For this review, take the finished solid that the model builds, in its own axes (mm). A direction names the side the tool comes from. Round coordinates to 2 decimals unless told otherwise and drop trailing zeros. Loops run counter-clockwise (first coordinate to the right, second up) from the corner with the lowest first, then second, coordinate; pieces in that order, holes last.
1) Insertion check: pin 1 (3 mm diameter, centred on y = 8, z = -0.5, fed in from +X); pin 2 (3 mm diameter, centred on x = 13.5, y = 3.5, fed in from -Z); pin 3 (8 mm diameter, centred on y = 15, z = -6, fed in from +X); pin 4 (1.5 mm diameter, centred on x = 1, y = 14, fed in from +Z). Each pin has a flat end and moves straight along its axis. Give the tip position at first contact, or say it passes through.
2) Take a section at B-B (z = 0). State the section outline as (x, y) points (3 decimals), then the cut area to 3 significant figures.
3) Take a section at C-C (y = 7.5). State the section outline as (x, z) points.
4) Wall thickness on L1, parallel to Y at x = 3.5, z = 7.25; L2, parallel to Y at x = 9.5, z = -3.25 (3 decimals); L3, parallel to X at y = 11.25, z = -1.75: over which ranges is each line inside the solid? List them lowest first.
5) Take a section at D-D (z = 2.5). State the section outline as (x, y) points (3 decimals).
6) Tool access review of faces 1 (the cylindrical face through (14.5, 5.5, 5)), 2 (the flat face through (16.5, 6, 5)), 3 (the cylindrical face through (7.62, 4.68, -3.16)), 4 (the flat face through (-4, 9.5, 0)), 5 (the cylindrical face through (14.5, 6.5, 5)): name each direction out of +Z, -Z, +X, -X, +Y, -Y from which nothing blocks a thin tool from reaching the whole face with its end or side.
7) Take a section at A-A (x = 0). State the section outline as (y, z) points.
Solid Edge part; units mm, degrees
sketch "Sketch1" plane through (0, 0, 0) normal (0, -1, 0) x (1, 0, 0)
  circle A0 centre (0, 0) radius 8.25
extrude "Protrusion1" add sketch "Sketch1" against normal blind 9.5
sketch "Sketch2" plane through (0, 9.5, 0) normal (0, 1, 0) x (0, 0, -1)
  circle A0 centre (0, 0) radius 3
extrude "ExtrudedProtrusion_2" add sketch "Sketch2" along normal blind 15
sketch "Sketch3" plane through (0, 6, 0) normal (0, 1, 0) x (0, 0, -1)
  line L0 (-7.62, -12.5) -> (-7.62, -3.162)
  line L1 (7.62, -3.162) -> (-7.62, -3.162)
  line L2 (7.62, -12.5) -> (7.62, -3.162)
  line L3 (5.5, -12.5) -> (7.62, -12.5)
  line L4 (5.5, -16.5) -> (5.5, -12.5)
  line L5 (4.5, -16.5) -> (5.5, -16.5)
  line L6 (4.5, -12.5) -> (4.5, -16.5)
  line L7 (0.5, -12.5) -> (4.5, -12.5)
  line L8 (0.5, -16.5) -> (0.5, -12.5)
  line L9 (-0.5, -16.5) -> (0.5, -16.5)
  line L10 (-0.5, -12.5) -> (-0.5, -16.5)
  line L11 (-4.5, -12.5) -> (-0.5, -12.5)
  line L12 (-4.5, -16.5) -> (-4.5, -12.5)
  line L13 (-5.5, -16.5) -> (-4.5, -16.5)
  line L14 (-5.5, -12.5) -> (-5.5, -16.5)
  line L15 (-5.5, -12.5) -> (-7.62, -12.5)
extrude "ExtrudedProtrusion_3" add sketch "Sketch3" along normal mid plane 0.25
sketch "Sketch4" plane through (16.5, 6, 5) normal (1, 0, 0) x (0, 0, -1)
  circle A0 centre (0, 0) radius 0.5
  circle A1 centre (5, 0) radius 0.5
  circle A2 centre (10, 0) radius 0.5
extrude "Protrusion2" add sketch "Sketch4" against normal up to vertex (4 mm away)
Response:
1. pin 1: stops at x = 8.25
1. pin 2: passes through
1. pin 3: stops at x = 2.24
1. pin 4: stops at z = 2.99
2. outline: (-8.25, 0) - (8.25, 0) - (8.25, 5.875) - (12.5, 5.875) - (12.5, 5.5) - (16.5, 5.5) - (16.5, 6.5) - (12.5, 6.5) - (12.5, 6.125) - (8.25, 6.125) - (8.25, 9.5) - (3, 9.5) - (3, 24.5) - (-3, 24.5) - (-3, 9.5) - (-8.25, 9.5) - close
2. area: 252 mm2
3. outline: circle Ø16.5 at (0, 0)
4. L1: y = 0 to 9.5
4. L2: y = 5.875 to 6.125
4. L3: x = -2.44 to 2.44
5. outline: (-7.862, 0) - (7.862, 0) - (7.862, 5.875) - (12.5, 5.875) - (12.5, 6.125) - (7.862, 6.125) - (7.862, 9.5) - (1.658, 9.5) - (1.658, 24.5) - (-1.658, 24.5) - (-1.658, 9.5) - (-7.862, 9.5) - close
6. face 1: +X, -Y
6. face 2: +Z, -Z, +X, +Y, -Y
6. face 3: none
6. face 4: +Y
6. face 5: +X, +Y
7. outline: (0, -8.25) - (9.5, -8.25) - (9.5, -3) - (24.5, -3) - (24.5, 3) - (9.5, 3) - (9.5, 8.25) - (0, 8.25) - close
